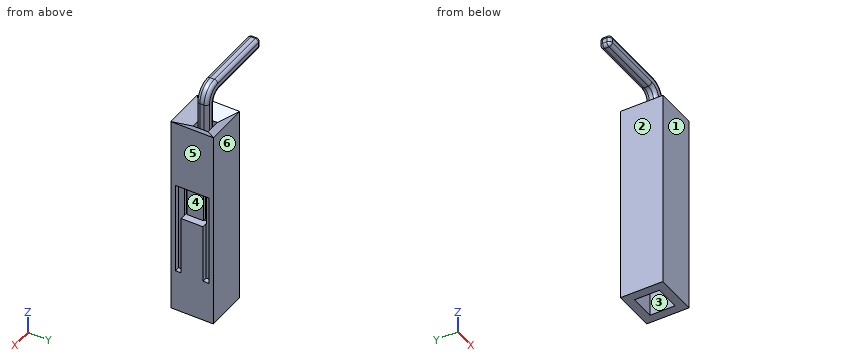
Autodesk Fusion 360 part; units mm, degrees
sketch "Sketch1" plane through (0, 0, 0) normal (0, 0, 1) x (1, 0, 0)
  line L0 (1.27, -1.27) -> (-1.27, -1.27)
  line L1 (-1.27, -1.27) -> (-1.27, 1.27)
  line L2 (-1.27, 1.27) -> (1.27, 1.27)
  line L3 (1.27, 1.27) -> (1.27, -1.27)
  line L4 (1.27, -1.27) -> (-1.27, 1.27) construction
  line L5 (-1.27, -1.27) -> (1.27, 1.27) construction
  dimension "d1" = 2.54
  dimension "d2" = 2.54
extrude "Extrude1" add sketch "Sketch1" along normal blind 12
sketch "Sketch2" plane through (0, 0, 12) normal (0, 0, 1) x (-1, 0, 0)
  line L0 (-1.27, -1.27) -> (1.27, -1.27)
  line L1 (1.27, -1.27) -> (1.27, 1.27)
  line L2 (1.27, 1.27) -> (-1.27, 1.27)
  line L3 (-1.27, 1.27) -> (-1.27, -1.27)
  line L4 (-0.45, 0.45) -> (0.45, 0.45)
  line L5 (0.45, 0.45) -> (0.45, -0.45)
  line L6 (0.45, -0.45) -> (-0.45, -0.45)
  line L7 (-0.45, -0.45) -> (-0.45, 0.45)
  line L8 (-0.45, 0.45) -> (0.45, -0.45) construction
  line L9 (0.45, 0.45) -> (-0.45, -0.45) construction
  dimension "d5" = 0.9
  dimension "d6" = 0.9
extrude "Extrude2" cut sketch "Sketch2" against normal blind 0.5 contours L4 L5 L6 L7
loft "Loft1" cut profiles "Sketch2" section 1 section 2 face at (0.15, -0.15, 11.5)
extrude "Extrude3" cut 1 faces at (0.15, -0.15, 11.5) along direction (0, 0, -1) blind 8
sketch "Sketch3" plane through (1.27, 0, 0) normal (1, 0, 0) x (0, 1, 0)
  line L0 (-1.27, 0) -> (1.27, 0)
  line L1 (1.27, 0) -> (1.27, 12)
  line L2 (1.27, 12) -> (-1.27, 12)
  line L3 (-1.27, 12) -> (-1.27, 0)
  line L4 (1, 8) -> (-1, 8)
  line L5 (-1, 8) -> (-1, 2.5)
  line L6 (-1, 2.5) -> (1, 2.5)
  line L7 (1, 2.5) -> (1, 8)
  line L8 (1, 8) -> (-1, 2.5) construction
  line L9 (-1, 8) -> (1, 2.5) construction
  line L10 (0.6482, 2.5061) -> (-0.6518, 2.5061)
  line L11 (-0.6518, 2.5061) -> (-0.6518, 6.0061)
  line L12 (-0.6518, 6.0061) -> (0.6482, 6.0061)
  line L13 (0.6482, 6.0061) -> (0.6482, 2.5061)
  line L14 (0.6482, 2.5061) -> (-0.6518, 6.0061) construction
  line L15 (-0.6518, 2.5061) -> (0.6482, 6.0061) construction
  line L16 (-0.6518, 6.0061) -> (0.6571, 6.0061)
  line L17 (0.6571, 6.0061) -> (0.6571, 8.0061)
  line L18 (0.6571, 8.0061) -> (-0.6518, 8.0061)
  line L19 (-0.6518, 8.0061) -> (-0.6518, 6.0061)
  line L20 (0.5, 6.1311) -> (-0.5, 6.1311)
  line L21 (-0.5, 6.1311) -> (-0.5, 7.8811)
  line L22 (-0.5, 7.8811) -> (0.5, 7.8811)
  line L23 (0.5, 7.8811) -> (0.5, 6.1311)
  line L24 (0.5, 6.1311) -> (-0.5, 7.8811) construction
  line L25 (-0.5, 6.1311) -> (0.5, 7.8811) construction
  line L26 (-1.27, 6) -> (-0.6518, 6.0061)
  line L27 (0.6571, 6.0061) -> (1.27, 6)
  line L28 (0.6482, 2.5061) -> (1, 2.5)
  line L29 (-0.6518, 2.5061) -> (-1, 2.5)
  point P0 (0, 5.25)
  point P1 (-0.0018, 4.2561)
  point P2 (0, 7.0061)
  dimension "d11" = 5.5
  dimension "d12" = 2.5
  dimension "d13" = 1.3
  dimension "d14" = 3.5
  dimension "d15" = 2
  dimension "d16" = 1
  dimension "d17" = 1.75
  dimension "d31" = 0.125
extrude "Extrude4" cut sketch "Sketch3" against normal blind 0.3 contours L5 L11 L26 L29 | L4 L5 L19 L26 | L4 L7 L17 L27 | L7 L13 L16 L27 L28
extrude "Extrude5" cut sketch "Sketch3" against normal blind 0.5 contours L4 L12 L16 L17 L19
extrude "Extrude6" cut sketch "Sketch3" against normal blind 0.3 contours L20 L21 L22 L23
sketch "Sketch4" plane through (0, 0, 0) normal (0, 0, -1) x (1, 0, 0)
  line L0 (-1.27, -1.27) -> (1.27, -1.27)
  line L1 (1.27, -1.27) -> (1.27, 1.27)
  line L2 (1.27, 1.27) -> (-1.27, 1.27)
  line L3 (-1.27, 1.27) -> (-1.27, -1.27)
  line L4 (0.75, -0.75) -> (-0.75, -0.75)
  line L5 (-0.75, -0.75) -> (-0.75, 0.75)
  line L6 (-0.75, 0.75) -> (0.75, 0.75)
  line L7 (0.75, 0.75) -> (0.75, -0.75)
  line L8 (0.75, -0.75) -> (-0.75, 0.75) construction
  line L9 (-0.75, -0.75) -> (0.75, 0.75) construction
  dimension "d24" = 1.5
  dimension "d25" = 1.5
extrude "Extrude7" cut sketch "Sketch4" against normal blind 2 contours L4 L5 L6 L7
sketch "Sketch5" plane through (0, 0, 2) normal (0, 0, -1) x (1, 0, 0)
  line L0 (0.75, 0.75) -> (-0.75, 0.75)
  line L1 (-0.75, 0.75) -> (-0.75, -0.75)
  line L2 (-0.75, -0.75) -> (0.75, -0.75)
  line L3 (0.75, -0.75) -> (0.75, 0.75)
  circle A0 centre (0, 0) radius 0.725
  dimension "d28" = 1.45
extrude "Extrude8" add sketch "Sketch5" along normal blind 0.1 contours A0
sketch "Sketch6" plane through (0, 0, 3.5) normal (0, 0, 1) x (-1, 0, 0)
  line L0 (-0.45, -0.45) -> (0.45, -0.45)
  line L1 (0.45, -0.45) -> (0.45, 0.45)
  line L2 (0.45, 0.45) -> (-0.45, 0.45)
  line L3 (-0.45, 0.45) -> (-0.45, -0.45)
  line L4 (-0.325, 0.325) -> (0.325, 0.325)
  line L5 (0.325, 0.325) -> (0.325, -0.325)
  line L6 (0.325, -0.325) -> (-0.325, -0.325)
  line L7 (-0.325, -0.325) -> (-0.325, 0.325)
  line L8 (-0.325, 0.325) -> (0.325, -0.325) construction
  line L9 (0.325, 0.325) -> (-0.325, -0.325) construction
  dimension "d32" = 0.65
  dimension "d33" = 0.65
extrude "Extrude9" add sketch "Sketch6" along normal blind 10.5 contours L4 L5 L6 L7
sketch "Sketch7" plane through (-0.325, 0, 0) normal (-1, 0, 0) x (0, -1, 0)
  line L0 (-0.325, 3.5) -> (0.325, 3.5)
  line L1 (0.325, 3.5) -> (0.325, 14)
  line L2 (0.325, 14) -> (-0.325, 14)
  line L3 (-0.325, 14) -> (-0.325, 3.5)
  line L4 (-0.325, 14) -> (0.325, 14)
  line L5 (0.325, 14) -> (0.325, 13.35)
  line L6 (0.325, 13.35) -> (-0.325, 13.35)
  line L7 (-0.325, 13.35) -> (-0.325, 14)
  dimension "d38" = 0.65
extrude "Extrude10" add sketch "Sketch7" along normal blind 4.5 contours L1 L2 L3 L4 L5 L6 L7
fillet "Fillet1" radius 0.2 12 edges at (0.325, -0.325, 8.75) (-0.325, -0.325, 8.425) (0.325, 0.325, 8.75) (-0.325, 0.325, 8.425) (-2.25, 0.325, 14) (-2.25, -0.325, 14) (-2.575, -0.325, 13.35) (-2.575, 0.325, 13.35) (-4.825, -0.325, 13.675) (-4.825, 0.325, 13.675) (-4.825, 0, 14) (-4.825, 0, 13.35)
fillet "Fillet1" radius 1 1 edges at (0.325, 0, 14)
fillet "Fillet1" radius 0.5 1 edges at (-0.325, 0, 13.35)
equation "d34 = 8.50 mm + 2 mm"
CAD build for the part. Positions are in the model's coordinates, mm. Face numbers are marked on the shaded views. A direction names the side the tool comes from. Coordinates: 2 decimals unless noted, no trailing zeros. Order: outer loops, then holes, each group sorted by start corner. A loop starts at its lowest first (then second) coordinate and runs counter-clockwise, first axis right, second up. Notation, with made-up numbers: (82, 9) - (113, 9) arc R22 cw to (113, 15) - close; hole circle Ø7 at (79.25, -21). An arc over 180 degrees is marked (long way). Answer in a Markdown table with one row per item.
1. Pull direction Y, two halves, no side cores. Call the marked faces 4, 5 and 6: +Y half, -Y half, draft (parallel to the pull), parting line (faces both ways), or undercut.
Answer:
| item | result |
|---|---|
| face 4 | undercut |
| face 5 | draft |
| face 6 | +Y half |
2. Slice it at D-D, the plane z = 12.5. List the corners of the cut face in (x, y) (3 decimals), then the cut area to 3 significant figures.
Answer:
| item | result |
|---|---|
| outline | (-0.325, -0.125) arc R0.2 ccw to (-0.125, -0.325) - (0.125, -0.325) arc R0.2 ccw to (0.325, -0.125) - (0.325, 0.125) arc R0.2 ccw to (0.125, 0.325) - (-0.125, 0.325) arc R0.2 ccw to (-0.325, 0.125) - close |
| area | 0.388 mm² |
3. Slice it at B-B, the plane z = 4. List the corners of the cut face in (x, y) (3 decimals).
Answer:
| item | result |
|---|---|
| outline | (-1.27, -1.27) - (1.27, -1.27) - (1.27, -1) - (0.97, -1) - (0.97, -0.652) - (1.27, -0.652) - (1.27, 0.648) - (0.97, 0.648) - (0.97, 1) - (1.27, 1) - (1.27, 1.27) - (-1.27, 1.27) - close; (-0.325, -0.125) arc R0.2 ccw to (-0.125, -0.325) - (0.125, -0.325) arc R0.2 ccw to (0.325, -0.125) - (0.325, 0.125) arc R0.2 ccw to (0.125, 0.325) - (-0.125, 0.325) arc R0.2 ccw to (-0.325, 0.125) - close; hole (-0.45, -0.45) - (0.45, -0.45) - (0.45, 0.45) - (-0.45, 0.45) - close |
4. Drill centre lines: L1, parallel to X at y = -0.4, z = 4.25; L2, parallel to Y at x = 0.25, z = 7; L3, parallel to X at y = 0.4, z = 3.25. Where is each one in solid material? Low to high. Write a range as from..to.
Answer:
| item | result |
|---|---|
| L1 | -1.27..-0.45, 0.45..1.27 |
| L2 | -1.27..-0.45, -0.28..0.28, 0.45..1.27 |
| L3 | -1.27..1.27 |
5. Slice it at A-A, the plane z = 7.75. List the corners of the cut face in (x, y) (3 decimals), then the cut area to 3 significant figures.
Answer:
| item | result |
|---|---|
| outline | (-1.27, -1.27) - (1.27, -1.27) - (1.27, -1) - (0.97, -1) - (0.97, -0.652) - (0.77, -0.652) - (0.77, -0.5) - (0.97, -0.5) - (0.97, 0.5) - (0.77, 0.5) - (0.77, 0.657) - (0.97, 0.657) - (0.97, 1) - (1.27, 1) - (1.27, 1.27) - (-1.27, 1.27) - close; (-0.325, -0.125) arc R0.2 ccw to (-0.125, -0.325) - (0.125, -0.325) arc R0.2 ccw to (0.325, -0.125) - (0.325, 0.125) arc R0.2 ccw to (0.125, 0.325) - (-0.125, 0.325) arc R0.2 ccw to (-0.325, 0.125) - close; hole (-0.45, -0.45) - (0.45, -0.45) - (0.45, 0.45) - (-0.45, 0.45) - close |
| area | 5.37 mm² |
6. 3-axis set-ups, long thin cutter, end or side, ignore diameter. For the marked faces 1, 2 and 3: which of +Z, -Z, +X, -X, +Y, -Y reach the whole face in a straight line?
Answer:
| item | result |
|---|---|
| face 1 | +Z, -Z, +X, -X, -Y |
| face 2 | -Z, -X, +Y, -Y |
| face 3 | -Z |
7. Flat gauge pin, fed straight in: P1, Ø1.5, axis at y = 0.5, z = 12, coming from the -X side. Where does the tip first touch, or does it go through?
Answer:
| item | result |
|---|---|
| P1 | x = -1.27 |
8. Slice it at C-C, the plane x = -1.5. List the corners of the cut face in (y, z) (3 decimals), then the cut area to 3 significant figures.
Answer:
| item | result |
|---|---|
| outline | (-0.325, 13.55) arc R0.2 ccw to (-0.125, 13.35) - (0.125, 13.35) arc R0.2 ccw to (0.325, 13.55) - (0.325, 13.8) arc R0.2 ccw to (0.125, 14) - (-0.125, 14) arc R0.2 ccw to (-0.325, 13.8) - close |
| area | 0.388 mm² |
